```python
from build123d import *

# Parameters (mm, degrees)
BOSS_EXTRUDE1_DEPTH = 1.6
SKETCH4_R           = 1.6
CUT_EXTRUDE1_DEPTH  = 1.6


with BuildPart() as part:
    # Sketch3 → Boss-Extrude1 (new body)
    with BuildSketch(Plane(origin=(0, 0, 0), x_dir=(1, 0, 0), z_dir=(0, 1, 0))):
        Polygon((-34.1, 26.65), (29.56, 26.65), (31.56, 24.65), (31.56, 13.7), (34.1, 11.16), (34.1, -22.11), (31.56, -24.65), (31.56, -26.65), (-34.1, -26.65), align=None)
    extrude(amount=BOSS_EXTRUDE1_DEPTH)

    # Sketch4 → Cut-Extrude1 (cut)
    with BuildSketch(Plane(origin=(0, 1.6, 0), x_dir=(1, 0, 0), z_dir=(0, 1, 0))):
        with Locations(Location((-19.1, 23.85, 0), (0, 0, 270))):
            Circle(SKETCH4_R)
        with Locations(Location((31.7, 8.65, 0), (0, 0, 270))):
            Circle(SKETCH4_R)
        with Locations(Location((31.7, -19.25, 0), (0, 0, 270))):
            Circle(SKETCH4_R)
        with Locations(Location((-20.2, -23.95, 0), (0, 0, 270))):
            Circle(SKETCH4_R)
    extrude(amount=-CUT_EXTRUDE1_DEPTH, mode=Mode.SUBTRACT)


solid = part.part
```
Check sheet for the modelled part. Datum: model origin and axes. Units: mm. A direction names the side the tool comes from. Round coordinates to 2 decimals unless told otherwise and drop trailing zeros. Order: outer loops, then holes, each group sorted by start corner. A loop starts at its lowest first (then second) coordinate and runs counter-clockwise, first axis right, second up. Notation, with made-up numbers: (51.25, 38.5) -> (103.25, 38.5) arc R19 ccw to (103.25, 62.5) -> close; hole circle Ø9 at (0.5, 82.25). An arc over 180 degrees is marked (long way). Use CSV: the item, a comma, the result in double quotes.
(1) Tool access check on faces 4 (the face through (31.56, 1, -19)), 5 (the face through (31.56, 1, 26)), 6 (the face through (-3, 1, -26.65)). Record the directions out of +Z, -Z, +X, -X, +Y, -Y that give a thin tool (end or side, any length) a straight path to the whole face; none if there is none.
Worked out:
face 4,"-Z, +X, +Y, -Y"
face 5,"+Z, +X, +Y, -Y"
face 6,"-Z, +X, -X, +Y, -Y"
(2) Cross-section at A-A (z = 19.25). Record the boundary of the cut face in (x, y), and give its area (3 significant figures).
Worked out:
outline,"(-34.1, 0) -> (30.1, 0) -> (30.1, 1.6) -> (-34.1, 1.6) -> close; (33.3, 0) -> (34.1, 0) -> (34.1, 1.6) -> (33.3, 1.6) -> close"
area,"104 mm²"
(3) Cross-section at B-B (y = 0.6). Record the boundary of the cut face in (x, z), and give its area (3 significant figures).
Worked out:
outline,"(-34.1, -26.65) -> (29.56, -26.65) -> (31.56, -24.65) -> (31.56, -13.7) -> (34.1, -11.16) -> (34.1, 22.11) -> (31.56, 24.65) -> (31.56, 26.65) -> (-34.1, 26.65) -> close; hole circle Ø3.2 at (-20.2, 23.95); hole circle Ø3.2 at (-19.1, -23.85); hole circle Ø3.2 at (31.7, -8.65); hole circle Ø3.2 at (31.7, 19.25)"
area,"3,560 mm²"
(4) Material ranges on line 1 along X through (y, z) = (0.95, -8.65); line 2 along X through (y, z) = (0.95, -23.85); line 3 along X through (y, z) = (1.35, -12.5), recorded low to high. Write a range as from..to.
Worked out:
line 1,"-34.1..30.1, 33.3..34.1"
line 2,"-34.1..-20.7, -17.5..31.56"
line 3,"-34.1..32.76"
(5) Cross-section at C-C (z = -23.85). Record the boundary of the cut face in (x, y), and give its area (3 significant figures).
Worked out:
outline,"(-34.1, 0) -> (-20.7, 0) -> (-20.7, 1.6) -> (-34.1, 1.6) -> close; (-17.5, 0) -> (31.56, 0) -> (31.56, 1.6) -> (-17.5, 1.6) -> close"
area,"99.9 mm²"
(6) Draft check along Z on faces 1 (the face through (-1, 1, 26.65)), 2 (the face through (30.7, 0.8, 18)), 3 (the face through (0, 0, 0)). Enter one of: pulls with the +Z half, pulls with the -Z half, needs draft (parallel to the pull), parting line crosses it, or undercut.
Worked out:
face 1,"pulls with the +Z half"
face 2,"undercut"
face 3,"needs draft"
